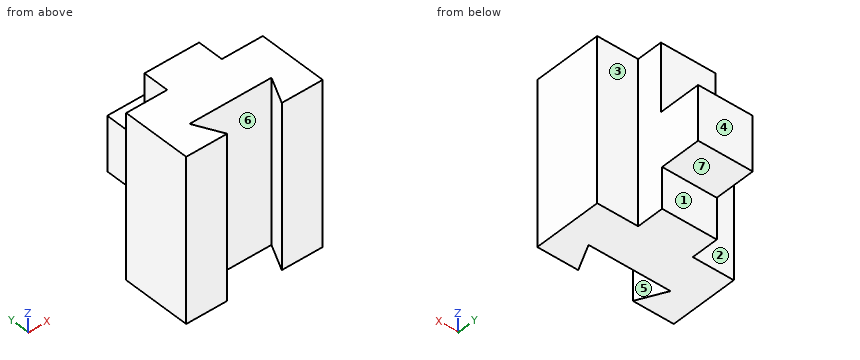
from build123d import *

# Parameters (mm, degrees)
IZIM1_W                     = 50
IZIM1_H                     = 50
Y_KSEKLIK_EKSTR_ZYON1_DEPTH = 60
KES_EKSTR_ZYON1_DEPTH       = 60
IZIM3_W                     = 15
IZIM3_H                     = 25
KES_EKSTR_ZYON2_DEPTH       = 60
IZIM4_W                     = 15
IZIM4_H                     = 15
IZIM4_W_2                   = 25
IZIM4_H_2                   = 15.532057861
KES_EKSTR_ZYON3_DEPTH       = 20


with BuildPart() as part:
    # Çizim1 → Yükseklik-Ekstrüzyon1 (new body)
    with BuildSketch(Plane.XY):
        with Locations((-13.102970675, -2.631578947)):
            Rectangle(IZIM1_W, IZIM1_H)
    extrude(amount=Y_KSEKLIK_EKSTR_ZYON1_DEPTH)

    # Çizim2 → Kes-Ekstrüzyon1 (cut)
    with BuildSketch(Plane.XY.offset(60)):
        Polygon((-28.102970675, -17.631578947), (1.897029325, -17.631578947), (-3.102970675, -27.631578947), (-23.102970675, -27.631578947), align=None)
    extrude(amount=-KES_EKSTR_ZYON1_DEPTH, mode=Mode.SUBTRACT)

    # Çizim3 → Kes-Ekstrüzyon2 (cut)
    with BuildSketch(Plane.XY.offset(60)):
        with Locations((4.397029325, 9.868421053)):
            Rectangle(IZIM3_W, IZIM3_H)
        with Locations((-30.602970675, 9.868421053)):
            Rectangle(IZIM3_W, IZIM3_H)
    extrude(amount=-KES_EKSTR_ZYON2_DEPTH, mode=Mode.SUBTRACT)

    # Çizim4 → Kes-Ekstrüzyon3 (cut)
    with BuildSketch(Plane.ZY.offset(23.102970675)):
        with Locations((7.5, 14.868421053)):
            Rectangle(IZIM4_W, IZIM4_H)
        with Locations((47.5, 14.602392123)):
            Rectangle(IZIM4_W_2, IZIM4_H_2)
    extrude(amount=-KES_EKSTR_ZYON3_DEPTH, mode=Mode.SUBTRACT)


solid = part.part
Geometry: final body of the model. Coordinates: model frame, mm. Face numbers are marked on the shaded views. A direction names the side the tool comes from. Round coordinates to 2 decimals unless told otherwise and drop trailing zeros. Order: outer loops, then holes, each group sorted by start corner. A loop starts at its lowest first (then second) coordinate and runs counter-clockwise, first axis right, second up. Notation, with made-up numbers: (-13.75, 7.25) - (21.25, 7.25) arc R18 ccw to (21.25, 41.25) - close; hole circle Ø8 at (39, 34.5). An arc over 180 degrees is marked (long way). Write each question's results on one line, items separated by ' | '.
Item 1: Material intervals for line 1 along Z through (x, y) = (-19, 10); line 2 along Y through (x, z) = (-5, 42.5); line 3 along Y through (x, z) = (-23, 29), sorted ascending. Write a range as [from, to].
Completed:
line 1: [15, 35] | line 2: [-17.63, 6.84] | line 3: [-17.63, 22.37]
Item 2: Section A-A, the plane z = 24. Return the cut outline in (x, y), and give its area (3 significant figures).
Completed:
outline: (-38.1, -27.63) - (-23.1, -27.63) - (-28.1, -17.63) - (1.9, -17.63) - (-3.1, -27.63) - (11.9, -27.63) - (11.9, -2.63) - (-3.1, -2.63) - (-3.1, 22.37) - (-23.1, 22.37) - (-23.1, -2.63) - (-38.1, -2.63) - close | area: 1,500 mm^2
Item 3: Reachability of the marked faces 1, 2 and 3 from +Z, -Z, +X, -X, +Y, -Y: full face, straight path, thin tool, end or side. Return the list, or none.
Completed:
face 1: -Z, +X, -X, +Y | face 2: +Z, -Z, -X, +Y | face 3: +Z, -Z, +X, +Y
Item 4: Section D-D, the plane z = 13.5. Return the cut outline in (x, y), and give its area (3 significant figures).
Completed:
outline: (-38.1, -27.63) - (-23.1, -27.63) - (-28.1, -17.63) - (1.9, -17.63) - (-3.1, -27.63) - (11.9, -27.63) - (11.9, -2.63) - (-3.1, -2.63) - (-3.1, 7.37) - (-23.1, 7.37) - (-23.1, -2.63) - (-38.1, -2.63) - close | area: 1,200 mm^2
Item 5: Section B-B, the plane y = -23.5. Return the cut outline in (x, z).
Completed:
outline: (-38.1, 0) - (-25.17, 0) - (-25.17, 60) - (-38.1, 60) - close; (-1.04, 0) - (11.9, 0) - (11.9, 60) - (-1.04, 60) - close
Item 6: Section C-C, the plane x = -13. Return the cut outline in (y, z), and give its area (3 significant figures).
Completed:
outline: (-17.63, 0) - (7.37, 0) - (7.37, 15) - (22.37, 15) - (22.37, 35) - (6.84, 35) - (6.84, 60) - (-17.63, 60) - close | area: 1,790 mm^2
Item 7: First-contact query: pin 1 Ø4.5 at (x, y) = (-11, 16.5) entering from +Z; pin 2 Ø1 at (x, z) = (-1.5, 30) entering from +Y; pin 3 Ø1.5 at (x, y) = (-6.5, 14) entering from -Z. Flat tips, straight axial feed; report the tip coordinate or a pass-through.
Completed:
pin 1: z = 35 | pin 2: y = -2.63 | pin 3: z = 15
Item 8: Mould query, pull axis Y, two halves, no side actions, for the marked faces 4, 5, 6 and 7. Classes: pulls with the +Y half, pulls with the -Y half, needs draft (parallel to the pull), parting line crosses it, or undercut.
Completed:
face 4: pulls with the +Y half | face 5: undercut | face 6: undercut | face 7: needs draft
